Drawing for the job (mm, zero at the part's lowest x, y, z). Give positions to 0.01 mm unless a question says otherwise; leave off trailing zeros. Loops run counter-clockwise (first coordinate to the right, second up) from the corner with the lowest first, then second, coordinate; pieces in that order, holes last. Notation, with made-up numbers: M 58,-29 L 116,-29 A11 ccw 116,-25 Z; hole C 87.5,43 d1. An arc over 180 degrees is marked long. Answer in a Markdown table with one row per item. Add a question column.
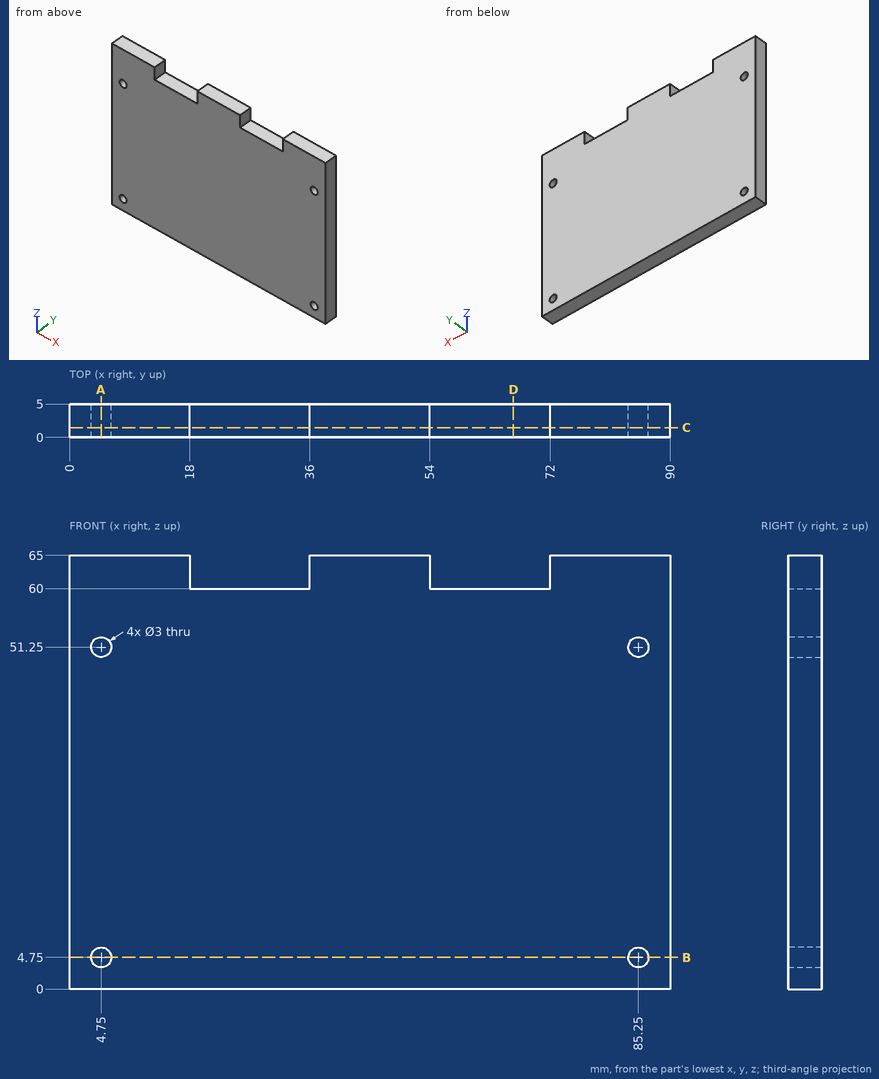
(1) Slice it at A-A, the plane x = 4.75. Give the cut face in (y, z), then the cut area to 3 significant figures.
(2) Pin check, flat tip, straight feed: pin 1 (2.5 mm diameter, centred on x = 66.5, y = 3, fed in from +Z). Stop position of the tip, or through.
(3) Slice it at B-B, the plane z = 4.75. Give the cut face in (x, y), then the cut area to 3 significant figures.
(4) Slice it at D-D, the plane x = 66.5. Give the cut face in (y, z), then the cut area to 3 significant figures.
(5) Slice it at C-C, the plane y = 1.45. Give the cut face in (x, z).
(6) Wall check: line 1 (X direction, y = 3.05, z = 4.75); line 2 (Z direction, x = 85.25, y = 3.15); line 3 (Z direction, x = 62.5, y = 4.05). Give the ranges that are in metal, low to high.
Solution:
| question | item | result |
|---|---|---|
| 1 | outline | M 0,0 L 5,0 L 5,3.25 L 0,3.25 Z; M 0,6.25 L 5,6.25 L 5,49.75 L 0,49.75 Z; M 0,52.75 L 5,52.75 L 5,65 L 0,65 Z |
| 1 | area | 295 mm^2 |
| 2 | pin 1 | z = 60 |
| 3 | outline | M 0,0 L 3.25,0 L 3.25,5 L 0,5 Z; M 6.25,0 L 83.75,0 L 83.75,5 L 6.25,5 Z; M 86.75,0 L 90,0 L 90,5 L 86.75,5 Z |
| 3 | area | 420 mm^2 |
| 4 | outline | M 0,0 L 5,0 L 5,60 L 0,60 Z |
| 4 | area | 300 mm^2 |
| 5 | outline | M 0,0 L 90,0 L 90,65 L 72,65 L 72,60 L 54,60 L 54,65 L 36,65 L 36,60 L 18,60 L 18,65 L 0,65 Z; hole C 4.75,4.75 d3; hole C 4.75,51.25 d3; hole C 85.25,4.75 d3; hole C 85.25,51.25 d3 |
| 6 | line 1 | 0 to 3.25, 6.25 to 83.75, 86.75 to 90 |
| 6 | line 2 | 0 to 3.25, 6.25 to 49.75, 52.75 to 65 |
| 6 | line 3 | 0 to 60 |
